CAD build for the part. Positions are in the model's coordinates, mm. A direction names the side the tool comes from. Give positions to 0.01 mm unless a question says otherwise; leave off trailing zeros. Write each loop counter-clockwise with the first axis right and the second up, starting at its lowest first coordinate (ties: lowest second). Pieces come first, ordered by that corner, then holes. Notation, with made-up numbers: (-23.5, 45) - (19.5, 45) arc R19 cw to (19.5, 61) - close; hole circle Ø5 at (88, -14.75). An arc over 180 degrees is marked (long way). Answer as a JSON object with one key per item and string values.
from build123d import *

# Parameters (mm, degrees)
F0_R     = 3.9385625542
F1_DEPTH = 50
F2_T     = -2.5


with BuildPart() as f1:
    # F0 (on Front) → F1 (new body)
    with BuildSketch(Plane.XZ):
        Polygon((-63.6753439903, 131.7894458771), (-110.7138618827, 71.7433527191), (-110.7138618827, -80.1898017526), (306.3688576221, -80.1898017526), (245.7079440355, 131.7894458771), align=None)
        with BuildLine():
            ThreePointArc((10.7150094085, 6.889880588), (12.6143743289, 3.0256211841), (13.267535524, -1.2303708618))
            ThreePointArc((13.267535524, -1.2303708618), (-5.1497771024, -14.7795789773), (-12.6024631263, 6.836061563))
            Line((-12.6024631263, 6.836061563), (-12.6024631263, 15.3979491442))
            Line((-12.6024631263, 15.3979491442), (10.7150094085, 15.3979491442))
            Line((10.7150094085, 15.3979491442), (10.7150094085, 6.889880588))
        make_face(mode=Mode.SUBTRACT)
        with Locations((89.6744132042, 11.8231130764)):
            Circle(F0_R, mode=Mode.SUBTRACT)
    extrude(amount=F1_DEPTH)

    # F2
    f2_openings = [f1.faces().sort_by_distance(p)[0] for p in [
        (86.977321, -50, 21.670217),
    ]]
    offset(amount=F2_T, openings=f2_openings, kind=Kind.INTERSECTION)


solid = f1.part
Item 1: Cut at A-A (y = -20). Give the cut face in (x, z) (3 decimals).
Entries:
{"outline": "(-110.714, -80.19) - (306.369, -80.19) - (245.708, 131.789) - (-63.675, 131.789) - (-110.714, 71.743) - close; (-15.102, 7.581) arc R16.693 ccw (long way) to (13.215, 7.641) - (13.215, 17.898) - (-15.102, 17.898) - close; circle Ø12.877 at (89.674, 11.823); hole (-108.214, -77.69) - (303.053, -77.69) - (243.823, 129.289) - (-62.458, 129.289) - (-108.214, 70.881) - close; hole (-12.602, 6.836) arc R14.193 ccw (long way) to (10.715, 6.89) - (10.715, 15.398) - (-12.602, 15.398) - close; hole circle Ø7.877 at (89.674, 11.823)"}
Item 2: Which spindle directions (+Z, -Z, +X, -X, +Y, -Y) get a long thin tool onto all of the face, cutting with end or side? Do faces 4 (the cylindrical face through (83.242, -25.918, 12.106)), 5 (the flat face through (276.46, -24.65, 24.32)), 6 (the flat face through (-1, -25, 15.398)). Say none if no direction does.
Entries:
{"face 4": "-Y", "face 5": "+Z, +X, +Y, -Y", "face 6": "+Y, -Y"}
Item 3: Mould opens along Z. For faces 1 (the flat face through (-13, -50, 7)), 2 (the flat face through (-1, -26, 17.898)), 3 (the flat face through (93, -25, 131.789)) say: +Z half, -Z half, draft (parallel to the pull), parting line (faces both ways), or undercut.
Entries:
{"face 1": "draft", "face 2": "undercut", "face 3": "+Z half"}
Item 4: Cut at D-D (z = -6.5). Give the cut face in (x, y).
Entries:
{"outline": "(-110.71, -50) - (-108.21, -50) - (-108.21, -2.5) - (-16.76, -2.5) - (-16.76, -50) - (-14.1, -50) - (-14.1, 0) - (-110.71, 0) - close; (12.25, -50) - (14.91, -50) - (14.91, -2.5) - (282.68, -2.5) - (282.68, -50) - (285.28, -50) - (285.28, 0) - (12.25, 0) - close"}
Item 5: Cut at C-C (z = -28.5). Give the cut face in (x, y).
Entries:
{"outline": "(-110.71, -50) - (-108.21, -50) - (-108.21, -2.5) - (288.98, -2.5) - (288.98, -50) - (291.58, -50) - (291.58, 0) - (-110.71, 0) - close"}
Item 6: Probe line 1 (Z direction, x = 100.5, y = -31.5); line 2 (Z direction, x = -8, y = -7.5); line 3 (X direction, y = -32.5, z = 11) (3 decimals). List the from-to ranges inside material, lowest first. Write a range as from..to.
Entries:
{"line 1": "-80.19..-77.69, 129.29..131.79", "line 2": "-80.19..-77.69, -16.35..-13.53, 15.4..17.9, 129.29..131.79", "line 3": "-110.714..-108.214, -15.102..-12.602, 10.715..13.215, 83.289..85.823, 93.526..96.06, 277.673..280.274"}
Item 7: Flat gauge pins, fed straight in: P1, Ø10, axis at x = 3, z = 84, coming from the -Y side; P2, Ø10, axis at y = -15.5, z = 103.5, coming from the -X side; P3, Ø11.5, axis at y = -30, z = 15, coming from the +X side. Where does each tip first touch, or does it go through?
Entries:
{"P1": "y = -2.5", "P2": "x = -89.75", "P3": "x = 280.77"}
Item 8: Cut at B-B (x = 237.5). Give the cut face in (y, z), and give its area (3 significant figures).
Entries:
{"outline": "(-50, -80.19) - (0, -80.19) - (0, 131.79) - (-50, 131.79) - (-50, 129.29) - (-2.5, 129.29) - (-2.5, -77.69) - (-50, -77.69) - close", "area": "767 mm2"}
